Autodesk Inventor part; units mm, degrees
ref_plane "YZ Plane" through (0, 0, 0) normal (1, 0, 0) x (0, 1, 0)
ref_plane "XZ Plane" through (0, 0, 0) normal (0, 1, 0) x (-1, 0, 0)
ref_plane "XY Plane" through (0, 0, 0) normal (0, 0, 1) x (1, 0, 0)
sketch "Szkic1" plane through (0, 0, 0) normal (0, 0, 1) x (1, 0, 0)
  circle A0 centre (0, 0) radius 3.5
  dimension "d0" = 7
extrude "Wyciągnięcie proste1" add sketch "Szkic1" along normal blind 4
chamfer "Faza1" distance 0.4 angle 45 1 edges at (-3.5, 0, 4)
sketch "Szkic2" plane through (0, 0, 4) normal (0, 0, 1) x (1, 0, 0)
  point P0 (0, 0)
sketch "Szkic3" plane through (0, 0, 4) normal (0, 0, 1) x (1, 0, 0)
  circle A0 centre (0, 0) radius 1.5355
  line L0 (1.5355, 0) -> (1.5355, 0.8865)
  line L1 (1.5355, 0) -> (1.5355, -0.8865)
  line L2 (0.7677, -1.3298) -> (1.5355, -0.8865)
  line L3 (0.7677, -1.3298) -> (0, -1.773)
  line L4 (0.7678, 1.3298) -> (0, 1.773)
  line L5 (-0.7677, 1.3298) -> (0, 1.773)
  line L6 (-1.5355, 0) -> (-1.5355, 0.8865)
  line L7 (-0.7677, 1.3298) -> (-1.5355, 0.8865)
  line L8 (-0.7678, -1.3298) -> (0, -1.773)
  line L9 (0.7678, 1.3298) -> (1.5355, 0.8865)
  line L10 (-1.5355, 0) -> (-1.5355, -0.8865)
  line L11 (-0.7678, -1.3298) -> (-1.5355, -0.8865)
  dimension "d6" = 3.071
extrude "Wyciągnięcie proste2" cut sketch "Szkic3" against normal blind 2
sketch "Szkic4" plane through (0, 0, 0) normal (0, 0, -1) x (-1, 0, 0)
  circle A0 centre (0, 0) radius 2
  dimension "d13" = 4
extrude "Wyciągnięcie proste3" add sketch "Szkic4" along normal blind 45
fillet "Zaokrąglenie1" radius 0.2 1 edges at (2, 0, 0)
sketch "Szkic5" plane through (0, 0, 0) normal (0, 0, -1) x (-1, 0, 0)
  point P0 (0, 0)
chamfer "Faza2" distance 0.3 angle 45 1 edges at (2, 0, -45)
sketch "Szkic6" plane through (0, 0, -45) normal (0, 0, -1) x (-1, 0, 0)
  point P0 (0, 0)
properties part number "sruba"
Part model, mm, in its own coordinate system. A direction names the side the tool comes from. Give positions to 0.01 mm unless a question says otherwise; leave off trailing zeros. Loops run counter-clockwise (first coordinate to the right, second up) from the corner with the lowest first, then second, coordinate; pieces in that order, holes last. Notation, with made-up numbers: M 37,80.25 L 94,80.25 A8 ccw 94,94.25 Z; hole C 74,55 d6. An arc over 180 degrees is marked long. Return JSON: item names as keys, results as strings.
1) 3-axis set-ups, long thin cutter, end or side, ignore diameter. For faces 4 (the face through (-1.536, 0, 3)), 5 (the face through (-2, -2, 0)), 6 (the face through (1.3, -1.3, 4)): which of +Z, -Z, +X, -X, +Y, -Y reach the whole face in a straight line?
Calculated:
{"face 4": "+Z", "face 5": "-Z", "face 6": "+Z, +X, -X, +Y, -Y"}
2) Saw through at B-B, the plane z = -13. List the corners of the cut face in (x, y).
Calculated:
{"outline": "C 0,0 d4"}
3) Saw through at C-C, the plane z = 1. List the corners of the cut face in (x, y), then the cut area to 3 significant figures.
Calculated:
{"outline": "C 0,0 d7", "area": "38.5 mm2"}
4) Pull direction X, two halves, no side cores. Call faces 1 (the face through (3.233, 1.341, 1.775)), 2 (the face through (1.536, 0, 3)), 3 (the face through (0, 0, -45)): released by +X, released by -X, zero draft, split by the parting line, or undercut.
Calculated:
{"face 1": "split by the parting line", "face 2": "undercut", "face 3": "zero draft"}
5) Flat gauge pins, fed straight in: pin 1 Ø4 at (x, z) = (-0.5, -15.5) entering from -Y; pin 2 Ø0.5 at (y, z) = (-0.5, 3.5) entering from +X; pin 3 Ø4 at (x, z) = (-2.5, -18.5) entering from -Y; pin 4 Ø1 at (x, y) = (-1.5, 1) entering from -Z. Where does each tip first touch, or does it go through?
Calculated:
{"pin 1": "stops at y = -2", "pin 2": "stops at x = 3.49", "pin 3": "stops at y = -1.94", "pin 4": "stops at z = -45"}
6) Drill centre lines: line 1 (Z direction, x = -3, y = 0); line 2 (Z direction, x = 1.25, y = 0); line 3 (X direction, y = 1, z = -25.5). Where is each one in solid material? Low to high.
Calculated:
{"line 1": "z = 0 to 4", "line 2": "z = -45 to 2", "line 3": "x = -1.73 to 1.73"}
7) Saw through at A-A, the plane y = 0. List the corners of the cut face in (x, z), then the cut area to 3 significant figures.
Calculated:
{"outline": "M -3.5,0 L -2.2,0 A0.2 cw -2,-0.2 L -2,-44.7 L -1.7,-45 L 1.7,-45 L 2,-44.7 L 2,-0.2 A0.2 cw 2.2,0 L 3.5,0 L 3.5,3.6 L 3.1,4 L 1.54,4 L 1.54,2 L -1.54,2 L -1.54,4 L -3.1,4 L -3.5,3.6 Z", "area": "202 mm2"}
